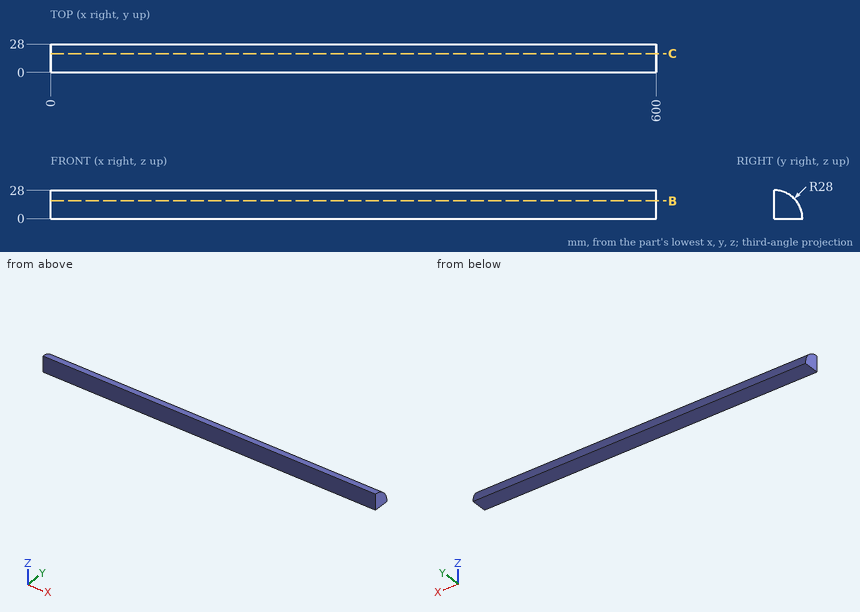
Print and shaded views of the part. All mm, measured from the part's lowest x, y and z. Coordinates: 2 decimals unless noted, no trailing zeros. Order: outer loops, then holes, each group sorted by start corner. A loop starts at its lowest first (then second) coordinate and runs counter-clockwise, first axis right, second up. Notation, with made-up numbers: (46.25, 39.5) - (64.25, 39.5) arc R12 cw to (64.25, 59.5) - close; hole circle Ø8 at (3.25, -30). An arc over 180 degrees is marked (long way). Return JSON: item names as keys, results as strings. Group by question number.
Item 1: Drill centre lines: probe 1 along Y at (x, z) = (152.5, 2.25); probe 2 along Y at (x, z) = (493, 1.5); probe 3 along Z at (x, y) = (267, 7.25) (3 decimals). Where is each one in solid material? Low to high. Write a range as from..to.
Item 2: Cut at C-C (y = 18.5). List the corners of the cut face in (x, z).
Item 3: Pin check, flat tips, straight feed: pin 1 (2 mm diameter, centred on x = 459.5, z = 6, fed in from +Y); pin 2 (1.5 mm diameter, centred on x = 129, y = 9.5, fed in from +Z). Stop position of each tip, or through.
Item 4: Cut at B-B (z = 17.5). List the corners of the cut face in (x, y).
Check values:
{
 "1": {"probe 1": "y = 0..27.91", "probe 2": "y = 0..27.96", "probe 3": "z = 0..27.045"},
 "2": {"outline": "(0, 0) - (600, 0) - (600, 21.02) - (0, 21.02) - close"},
 "3": {"pin 1": "stops at y = 27.55", "pin 2": "stops at z = 26.6"},
 "4": {"outline": "(0, 0) - (600, 0) - (600, 21.86) - (0, 21.86) - close"}
}
